```python
from build123d import *

# Parameters (mm, degrees)
SKETCH1_W           = 45
SKETCH1_H           = 25
SKETCH1_H_2         = 2
BOSS_EXTRUDE3_DEPTH = 2
SKETCH6_W           = 45
SKETCH6_H           = 2
BOSS_EXTRUDE4_DEPTH = 15
SKETCH7_R           = 1
CUT_EXTRUDE1_DEPTH  = 18
SKETCH9_R           = 1
SKETCH9_R_2         = 1.144474258
CUT_EXTRUDE3_DEPTH  = 18
SCALE1_SCALE        = 0.75


with BuildPart() as part:
    # Sketch1 → Boss-Extrude3 (new body)
    with BuildSketch(Plane.XY):
        Rectangle(SKETCH1_W, SKETCH1_H)
        with Locations((0, -13.5)):
            Rectangle(SKETCH1_W, SKETCH1_H_2)
    extrude(amount=BOSS_EXTRUDE3_DEPTH)

    # Sketch6 → Boss-Extrude4 (add)
    with BuildSketch(Plane.XY.offset(2)):
        with Locations((0, -13.5)):
            Rectangle(SKETCH6_W, SKETCH6_H)
    extrude(amount=-BOSS_EXTRUDE4_DEPTH)

    # Sketch7 → Cut-Extrude1 (cut)
    with BuildSketch(Plane(origin=(0, 0, 0), x_dir=(-1, 0, 0), z_dir=(0, 0, -1))):
        with Locations((-20, 10)):
            Circle(SKETCH7_R)
        with Locations((20, -5)):
            Circle(SKETCH7_R)
    extrude(amount=-CUT_EXTRUDE1_DEPTH, mode=Mode.SUBTRACT)

    # Sketch9 → Cut-Extrude3 (cut)
    with BuildSketch(Plane(origin=(0, -12.5, 0), x_dir=(1, 0, 0), z_dir=(0, 1, 0))):
        with Locations(Location((-18.5, 7, 0), (0, 0, 180))):
            Circle(SKETCH9_R)
        with Locations(Location((18.5, 7, 0), (0, 0, 180))):
            Circle(SKETCH9_R_2)
    extrude(amount=-CUT_EXTRUDE3_DEPTH, mode=Mode.SUBTRACT)


with BuildPart() as part_1:
    # Scale1: scaled about (-0.010079513, -5.05482545, -1.423478353)
    add(part.part.scale(SCALE1_SCALE).moved(Location((-0.002519878, -1.263706363, -0.355869588))))


solid = part_1.part
```
Read the model definition and answer for the solid it produces. Units are mm, in the model's axes. A direction names the side the tool comes from. Coordinates: 2 decimals unless noted, no trailing zeros. Write each loop counter-clockwise with the first axis right and the second up, starting at its lowest first coordinate (ties: lowest second). Pieces come first, ordered by that corner, then holes. Notation, with made-up numbers: (81.5, -39) - (87.5, -39) arc R27 cw to (87.5, -1) - close; hole circle Ø6 at (15, 25). An arc over 180 degrees is marked (long way). Answer as a JSON object with one key per item and string values. Group by question number.
1. Consider L1, parallel to Y at x = 8.5, z = -6.5; L2, parallel to Z at x = 7, y = -9.75. Determine where each line is inside the solid, lowest interval first. Write a range as [from, to].
2. Each of these flat-tipped pins is pushed along its axis until it touches: P1, Ø1, axis at x = 10.5, z = -1, coming from the +Y side; P2, Ø1.4, axis at x = 15, y = 6.24, coming from the +Z side; P3, Ø9.5, axis at x = -6, y = -2, coming from the -Z side. Where does it stop, or does it pass through?
3. Which of the six approach directions +Z, -Z, +X, -X, +Y, -Y give full straight-line access (tool end or side, diameter ignored) to faces 4 (the flat face through (0, -12.139, -4)), 5 (the flat face through (0, -1, -0.356))?
4. A cutting plane is placed at B-B (y = -9.5). Determine the outline of the cut face in (x, z), plus the area to 3 significant figures.
5. A cutting plane is placed at A-A (x = 11.5). Determine the outline of the cut face in (y, z).
6. A cutting plane is placed at C-C (z = -3.5). Determine the outline of the cut face in (x, y).
7. The mould has two halves that part along X. Classify faces 1 (the flat face through (0, -2, 1.144)), 2 (the cylindrical face through (-14.6, -11.4, -5.4)), 3 (the flat face through (16.872, -5, 0)): +X half, -X half, draft (parallel to the pull), parting line (faces both ways), or undercut.
Worked out:
{
 "1": {"L1": "y = [-12.14, -10.64]", "L2": "z = [-0.36, 1.14]"},
 "2": {"P1": "stops at y = -10.64", "P2": "passes through", "P3": "stops at z = -0.36"},
 "3": {"face 4": "+Z, -Z, +X, -X, -Y", "face 5": "-Z, +X, -X, +Y"},
 "4": {"outline": "(-16.88, -0.36) - (16.87, -0.36) - (16.87, 1.14) - (-16.88, 1.14) - close", "area": "50.6 mm²"},
 "5": {"outline": "(-12.14, -10.11) - (-10.64, -10.11) - (-10.64, -0.36) - (8.11, -0.36) - (8.11, 1.14) - (-12.14, 1.14) - close"},
 "6": {"outline": "(-16.88, -12.14) - (16.87, -12.14) - (16.87, -10.64) - (-16.88, -10.64) - close"},
 "7": {"face 1": "draft", "face 2": "undercut", "face 3": "+X half"}
}
